```python
from build123d import *

# Parameters (mm, degrees)
CROQUIS1_W  = 52
CROQUIS1_H  = 2.5
REDONDEO1_R = 0.25


with BuildPart() as part:
    # Croquis1 → Revolución1 (revolve)
    with BuildSketch(Plane.XY):
        with Locations((26, 1.25)):
            Rectangle(CROQUIS1_W, CROQUIS1_H)
    revolve(axis=Axis((0, 0, 0), (1, 0, 0)))

    # Redondeo1
    redondeo1_edges = [part.edges().sort_by_distance(p)[0] for p in [
        (52, -2.5, 0),
    ]]
    fillet(redondeo1_edges, radius=REDONDEO1_R)

    # Croquis3 → Cortar-Revolución1 (revolve, cut)
    with BuildSketch(Plane.XY):
        Polygon((52, 0), (51.5, 0), (52, 1), align=None)
    revolve(axis=Axis((52, 0, 0), (-1, 0, 0)), mode=Mode.SUBTRACT)


solid = part.part
```
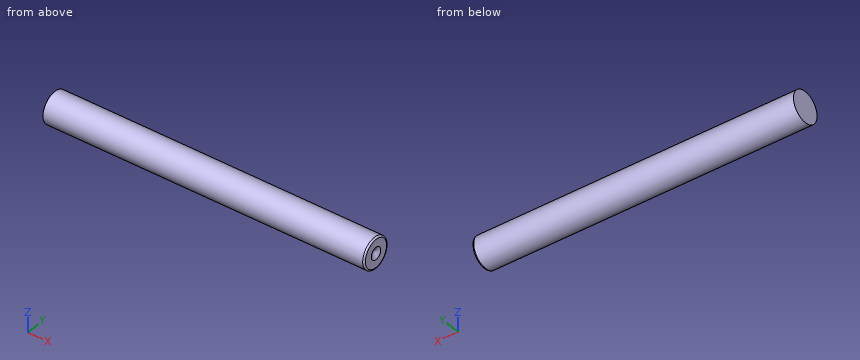
CAD build for the part. Positions are in the model's coordinates, mm. Round coordinates to 2 decimals unless told otherwise and drop trailing zeros. Write each loop counter-clockwise with the first axis right and the second up, starting at its lowest first coordinate (ties: lowest second). Pieces come first, ordered by that corner, then holes. Notation, with made-up numbers: (17, 70.5) -> (68, 70.5) arc R20 cw to (68, 92.5) -> close; hole circle Ø4 at (-33, -10.5). An arc over 180 degrees is marked (long way). Answer in a Markdown table with one row per item. Add a question column.
Item 1: Drill centre lines: line 1 (Y direction, x = 23.5, z = 0.1); line 2 (Y direction, x = 11.5, z = -0.9). Where is each one in solid material? Low to high. Write a range as from..to.
Item 2: Drop flat-ended pins along their axis: pin 1 Ø2 at (x, z) = (28, -2) entering from -Y; pin 2 Ø2 at (x, y) = (21.5, 1.5) entering from +Z. Give the stop position or say it passes through.
Item 3: Saw through at A-A, the plane x = 16. Write the cut outline in (y, z), then the cut area to 3 significant figures.
Findings below:
| question | item | result |
|---|---|---|
| 1 | line 1 | y = -2.5..2.5 |
| 1 | line 2 | y = -2.33..2.33 |
| 2 | pin 1 | stops at y = -2.29 |
| 2 | pin 2 | stops at z = 2.45 |
| 3 | outline | circle Ø5 at (0, 0) |
| 3 | area | 19.6 mm^2 |
